Build history of the part. All positions in model axes, mm. A direction names the side the tool comes from. Round coordinates to 2 decimals unless told otherwise and drop trailing zeros. Order: outer loops, then holes, each group sorted by start corner. A loop starts at its lowest first (then second) coordinate and runs counter-clockwise, first axis right, second up. Notation, with made-up numbers: (80.25, 60) - (104.25, 60) arc R36 ccw to (104.25, 97) - close; hole circle Ø2 at (55, 56.25). An arc over 180 degrees is marked (long way). One line per question, with ' | ' between items. Start each with the question number.
from build123d import *

# Parameters (mm, degrees)
F1_DEPTH = 30
F2_DEPTH = 20
F3_DEPTH = 10


with BuildPart() as f1:
    # F0 (on Front) → F1 (new body)
    with BuildSketch(Plane.XZ):
        Polygon((0, 10), (0, 0), (50, 0), (37.666667, 10), align=None)
        Polygon((37.666667, 10), (50, 0), (50, 30), (13, 30), (25.333333, 20), align=None)
        Polygon((0, 20), (0, 10), (37.666667, 10), (25.333333, 20), align=None)
        Polygon((0, 30), (0, 20), (25.333333, 20), (13, 30), align=None)
    extrude(amount=-F1_DEPTH)

    # F0 (on Front) → F2 (cut)
    with BuildSketch(Plane.XZ):
        Polygon((37.666667, 10), (50, 0), (50, 30), (13, 30), (25.333333, 20), align=None)
    extrude(amount=-F2_DEPTH, mode=Mode.SUBTRACT)

    # F0 (on Front) → F3 (cut)
    with BuildSketch(Plane.XZ):
        Polygon((0, 20), (0, 10), (37.666667, 10), (25.333333, 20), align=None)
    extrude(amount=-F3_DEPTH, mode=Mode.SUBTRACT)


solid = f1.part
Item 1: Pin check, flat tips, straight feed: pin 1 (3 mm diameter, centred on x = 28, z = 16.5, fed in from -Y); pin 2 (5 mm diameter, centred on y = 12, z = 11.5, fed in from +X); pin 3 (3 mm diameter, centred on x = 16, y = 7, fed in from +Z). Stop position of each tip, or through.
Item 2: Slice it at A-A (y = 5.75). Write the cut outline in (x, z).
Item 3: Pull direction Z, two halves, no side cores. Call faces 1 (the face through (20, 21, 30)), 2 (the face through (0, 15, 15)), 3 (the face through (13, 5, 20)): released by +Z, released by -Z, zero draft, split by the parting line, or undercut.
Item 4: Wall check: line 1 along Y through (x, z) = (46, 24.5); line 2 along X through (y, z) = (14, 20); line 3 along Z through (x, y) = (34, 1.5). Give the ranges that are in metal, low to high. Write a range as [from, to].
Item 5: Slice it at D-D (z = 25.75). Write the cut outline in (x, y), plus the area to 3 significant figures.
Item 6: Slice it at C-C (y = 18.5). Write the cut outline in (x, z).
Item 7: 3-axis set-ups, long thin cutter, end or side, ignore diameter. For faces 4 (the face through (10, 0, 25)), 5 (the face through (35, 20, 22)), 6 (the face through (19, 5, 10)): which of +Z, -Z, +X, -X, +Y, -Y reach the whole face in a straight line?
Item 8: Slice it at B-B (x = 9.5). Write the cut outline in (y, z), plus the area to 3 significant figures.
A:
1) pin 1: y = 10 | pin 2: x = 38.9 | pin 3: z = 28.78
2) outline: (0, 0) - (50, 0) - (37.67, 10) - (0, 10) - close; (0, 20) - (25.33, 20) - (13, 30) - (0, 30) - close
3) face 1: released by +Z | face 2: zero draft | face 3: undercut
4) line 1: [20, 30] | line 2: [0, 25.33] | line 3: [0, 10]
5) outline: (0, 0) - (18.24, 0) - (18.24, 20) - (50, 20) - (50, 30) - (0, 30) - close | area: 865 mm^2
6) outline: (0, 0) - (50, 0) - (13, 30) - (0, 30) - close
7) face 4: +Z, -Z, +X, -X, -Y | face 5: +Z, +X, -Y | face 6: +X, -X, -Y
8) outline: (0, 0) - (30, 0) - (30, 30) - (0, 30) - (0, 20) - (10, 20) - (10, 10) - (0, 10) - close | area: 800 mm^2
